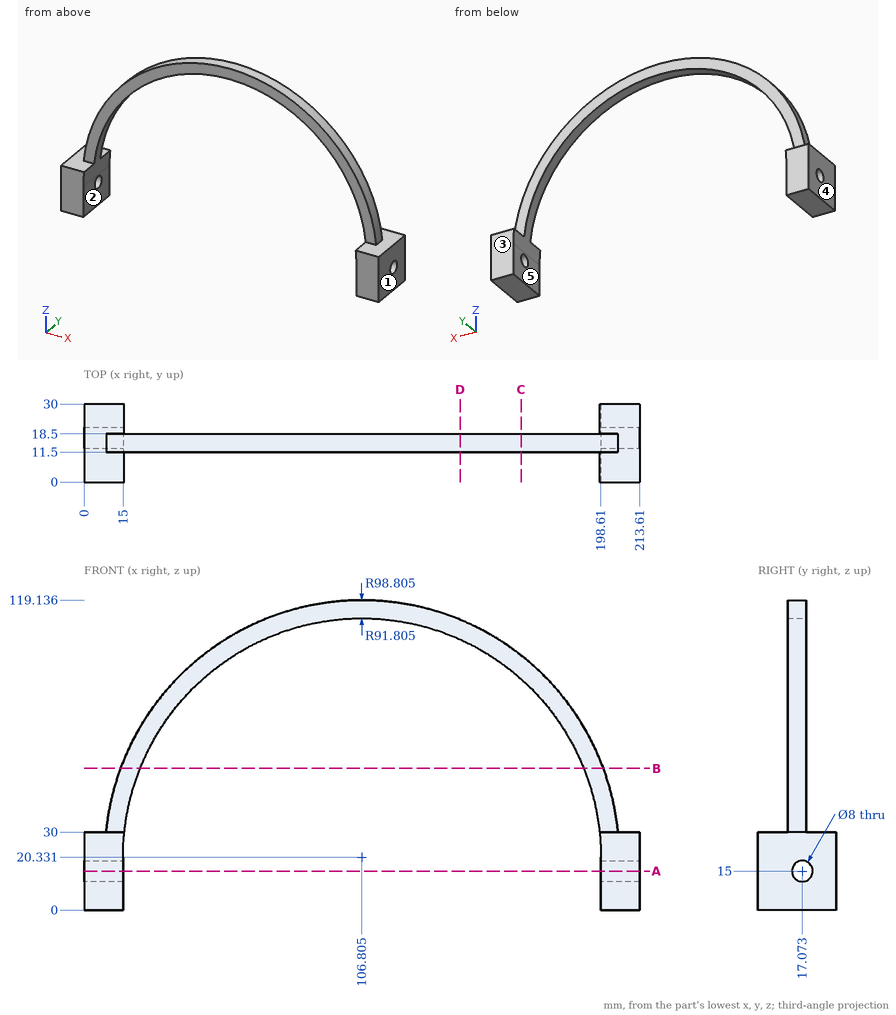
Design review of the part shown in the three views and the two pictorial views. Dimensions are in mm from the part's minimum x, y and z. A direction names the side the tool comes from. Give positions to 0.01 mm unless a question says otherwise; leave off trailing zeros. Loops run counter-clockwise (first coordinate to the right, second up) from the corner with the lowest first, then second, coordinate; pieces in that order, holes last. Notation, with made-up numbers: (64.25, 56) - (122.25, 56) arc R27 ccw to (122.25, 86) - close; hole circle Ø8 at (-1, 81). An arc over 180 degrees is marked (long way). Answer as a JSON object with one key per item and string values.
Q1. Add section C-C on x = 168. State the section outline as (y, z) points, plus the area to 3 significant figures.
Worked out:
{"outline": "(11.5, 88.77) - (18.5, 88.77) - (18.5, 97.9) - (11.5, 97.9) - close", "area": "64.0 mm^2"}
Q2. To check wall thickness, follow line 1 along X through (y, z) = (21.75, 10.5); line 2 along Y through (x, z) = (5.5, 15); line 3 along Z through (x, y) = (9, 4.5). State the ranges of each line that lie inside material, in increasing order.
Worked out:
{"line 1": "x = 0 to 15, 198.61 to 213.61", "line 2": "y = 0 to 13.07, 21.07 to 30", "line 3": "z = 0 to 30"}
Q3. Add section D-D on x = 144.5. State the section outline as (y, z) points.
Worked out:
{"outline": "(11.5, 104.04) - (18.5, 104.04) - (18.5, 111.66) - (11.5, 111.66) - close"}
Q4. Add section B-B on z = 54.5. State the section outline as (x, y) points.
Worked out:
{"outline": "(14.1, 11.5) - (21.6, 11.5) - (21.6, 18.5) - (14.1, 18.5) - close; (192.01, 11.5) - (199.51, 11.5) - (199.51, 18.5) - (192.01, 18.5) - close"}
Q5. Mouldability with a two-part tool opening along X and no side actions: class the marked faces 3, 4 and 5 as +X half, -X half, draft (parallel to the pull), parting line (faces both ways), or undercut.
Worked out:
{"face 3": "draft", "face 4": "-X half", "face 5": "undercut"}
Q6. Insertion check: pin 1 (8 mm diameter, centred on x = 202.5, y = 15, fed in from +Z) (1 decimal); pin 2 (4.5 mm diameter, centred on x = 4, y = 17, fed in from +Z); pin 3 (1.5 mm diameter, centred on x = 70.5, y = 18.5, fed in from -Z) (1 decimal). Each pin has a flat end and moves straight along its axis. Give the tip position at first contact, or say it passes through.
Worked out:
{"pin 1": "stops at z = 57.1", "pin 2": "stops at z = 30", "pin 3": "stops at z = 104.3"}
Q7. Add section A-A on z = 15. State the section outline as (x, y) points.
Worked out:
{"outline": "(0, 0) - (15, 0) - (15, 13.07) - (0, 13.07) - close; (0, 21.07) - (15, 21.07) - (15, 30) - (0, 30) - close; (198.61, 0) - (213.61, 0) - (213.61, 13.07) - (198.61, 13.07) - close; (198.61, 21.07) - (213.61, 21.07) - (213.61, 30) - (198.61, 30) - close"}
Q8. For the marked faces 1 and 2, list the 3-axis set-ups (+Z, -Z, +X, -X, +Y, -Y) from which the entire face can be reached by the end or side of a thin tool; tool diameter is ignored.
Worked out:
{"face 1": "+Z, -Z, +X, +Y, -Y", "face 2": "-Z, +Y, -Y"}
